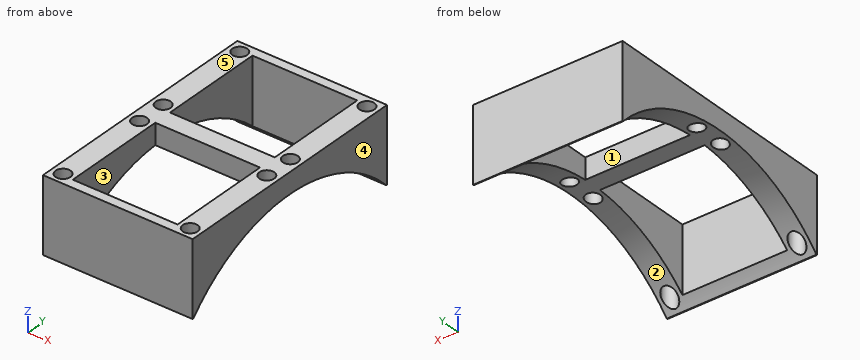
```python
from build123d import *

# Parameters (mm, degrees)
SKETCH1_W               = 40
SKETCH1_H               = 66
SKETCH1_W_2             = 28
SKETCH1_H_2             = 28
BOSS_EXTRUDE1_DEPTH     = 20
CUT_EXTRUDE1_DEPTH      = 26
CUT_EXTRUDE1_DEPTH_BACK = 27
SKETCH3_R               = 44.45
SKETCH4_R               = 2
CUT_EXTRUDE2_DEPTH      = 27
SKETCH5_R               = 2
CUT_EXTRUDE3_DEPTH      = 44.462627716


with BuildPart() as part:
    # Sketch1 → Boss-Extrude1 (new body)
    with BuildSketch(Plane.XY):
        Rectangle(SKETCH1_W, SKETCH1_H)
        with Locations((0, 16.5)):
            Rectangle(SKETCH1_W_2, SKETCH1_H_2, mode=Mode.SUBTRACT)
        with Locations((0, -16.5)):
            Rectangle(SKETCH1_W_2, SKETCH1_H_2, mode=Mode.SUBTRACT)
    extrude(amount=BOSS_EXTRUDE1_DEPTH)

    # Sketch3 → Cut-Extrude1 (cut, two sides: drawn at the far end of the back side and taken through both)
    with BuildSketch(Plane(origin=(0, 0, 0), x_dir=(0, 0, -1), z_dir=(1, 0, 0)).offset(-CUT_EXTRUDE1_DEPTH_BACK)):
        with Locations((30, 0)):
            Circle(SKETCH3_R)
    extrude(amount=CUT_EXTRUDE1_DEPTH + CUT_EXTRUDE1_DEPTH_BACK, mode=Mode.SUBTRACT)

    # Sketch4 → Cut-Extrude2 (cut)
    with BuildSketch(Plane.XY.offset(20)):
        with Locations((-17, 30)):
            Circle(SKETCH4_R)
        with Locations((17, 30)):
            Circle(SKETCH4_R)
        with Locations((-17, -30)):
            Circle(SKETCH4_R)
        with Locations((17, -30)):
            Circle(SKETCH4_R)
    extrude(amount=-CUT_EXTRUDE2_DEPTH, mode=Mode.SUBTRACT)

    # Sketch5 → Cut-Extrude3 (cut, through all)
    with BuildSketch(Plane.XY.offset(20)):
        with Locations((-17, 4)):
            Circle(SKETCH5_R)
        with Locations((-17, -4)):
            Circle(SKETCH5_R)
        with Locations((17, 4)):
            Circle(SKETCH5_R)
        with Locations((17, -4)):
            Circle(SKETCH5_R)
    extrude(amount=-CUT_EXTRUDE3_DEPTH, mode=Mode.SUBTRACT)


solid = part.part
```
The model under review builds one solid part; all positions refer to its coordinate system, in mm. Face numbers are marked on the shaded views. A direction names the side the tool comes from. Give positions to 0.01 mm unless a question says otherwise; leave off trailing zeros. Write each loop counter-clockwise with the first axis right and the second up, starting at its lowest first coordinate (ties: lowest second). Pieces come first, ordered by that corner, then holes. Notation, with made-up numbers: (49.25, -38) - (85.25, -38) arc R17 cw to (85.25, -22) - close; hole circle Ø1 at (21.25, 70). An arc over 180 degrees is marked (long way). Answer in a Markdown table with one row per item. Add a question column.
1. We need section B-B on z = 11.25. Write out the cut boundary in (x, y).
2. We need section C-C on y = -21.5. Write out the cut boundary in (x, z), then the cut area to 3 significant figures.
3. Tool access review of the marked faces 1 and 2: name each direction out of +Z, -Z, +X, -X, +Y, -Y from which nothing blocks a thin tool from reaching the whole face with its end or side.
4. We need section D-D on x = -17. Write out the cut boundary in (y, z).
5. Insertion check: P1, Ø8, axis at x = 2, y = 4, coming from the -Z side. The pin has a flat end and moves straight along its axis. Give the tip position at first contact, or say it passes through.
6. Draft analysis for pull direction X (two halves, no side actions). For the marked faces 3, 4 and 5, state which applies: +X half, -X half, draft (parallel to the pull), parting line (faces both ways), or undercut.
7. Wall thickness on line 1 along Y through (x, z) = (17, 17.15); line 2 along Y through (x, z) = (5.5, 16); line 3 along X through (y, z) = (30, 8.5): over which ranges is each line inside the solid? List them lowest first. Write a range as [from, to].
8. We need section A-A on x = -11.5. Write out the cut boundary in (y, z) (3 decimals).
Ans:
| question | item | result |
|---|---|---|
| 1 | outline | (-20, -33) - (20, -33) - (20, -16.56) - (14, -16.56) - (14, -30.5) - (-14, -30.5) - (-14, -16.56) - (-20, -16.56) - close; (-20, 16.56) - (-14, 16.56) - (-14, 30.5) - (14, 30.5) - (14, 16.56) - (20, 16.56) - (20, 33) - (-20, 33) - close; hole circle Ø4 at (-17, -30); hole circle Ø4 at (-17, 30); hole circle Ø4 at (17, -30); hole circle Ø4 at (17, 30) |
| 2 | outline | (-20, 8.9) - (-14, 8.9) - (-14, 20) - (-20, 20) - close; (14, 8.9) - (20, 8.9) - (20, 20) - (14, 20) - close |
| 2 | area | 133 mm^2 |
| 3 | face 1 | +Z, -Z |
| 3 | face 2 | -Z, +X, -X |
| 4 | outline | (-33, 0) - (-32.8, 0) arc R44.45 cw to (-32, 0.85) - (-32, 20) - (-33, 20) - close; (-28, 4.52) arc R44.45 cw to (-6, 14.04) - (-6, 20) - (-28, 20) - close; (-2, 14.4) arc R44.45 cw to (2, 14.4) - (2, 20) - (-2, 20) - close; (6, 14.04) arc R44.45 cw to (28, 4.52) - (28, 20) - (6, 20) - close; (32, 0.85) arc R44.45 cw to (32.8, 0) - (33, 0) - (33, 20) - (32, 20) - close |
| 5 | P1 | stops at z = 14.38 |
| 6 | face 3 | undercut |
| 6 | face 4 | +X half |
| 6 | face 5 | draft |
| 7 | line 1 | y = [-33, -32], [-28, -6], [-2, 2], [6, 28], [32, 33] |
| 7 | line 2 | y = [-33, -30.5], [-2.5, 2.5], [30.5, 33] |
| 7 | line 3 | x = [-20, -19], [-15, -14], [14, 15], [19, 20] |
| 8 | outline | (-33, 0) - (-32.799, 0) arc R44.45 cw to (-30.5, 2.335) - (-30.5, 20) - (-33, 20) - close; (-2.5, 14.38) arc R44.45 cw to (2.5, 14.38) - (2.5, 20) - (-2.5, 20) - close; (30.5, 2.335) arc R44.45 cw to (32.799, 0) - (33, 0) - (33, 20) - (30.5, 20) - close |
